Part model, mm, in its own coordinate system. Face numbers are marked on the shaded views. Coordinates: 2 decimals unless noted, no trailing zeros. Order: outer loops, then holes, each group sorted by start corner. A loop starts at its lowest first (then second) coordinate and runs counter-clockwise, first axis right, second up.
1) Cut at C-C (z = 6). List the corners of the cut face in (x, y), and give its area (3 significant figures).
2) Wall check: L1, parallel to Y at x = -13.25, z = 13; L2, parallel to X at y = 0, z = 9.5; L3, parallel to X at y = 1.5, z = 3. Give the ranges that are in metal, low to high.
3) Cut at A-A (x = -25.25). List the corners of the cut face in (y, z).
4) Cut at D-D (x = -12.25). List the corners of the cut face in (y, z).
5) Cut at B-B (z = 0.5). List the corners of the cut face in (x, y).
6) Mould opens along X. For the marked faces 1, 2 and 3 say: +X half, -X half, draft (parallel to the pull), parting line (faces both ways), or undercut.
7) Pin check, flat tips, straight feed: pin 1 Ø1 at (x, z) = (-10, 6.5) entering from -Y; pin 2 Ø6 at (x, y) = (-22.5, 7) entering from -Z; pin 3 Ø1 at (y, z) = (-4, -2) entering from -X. Stop position of each tip, or through.
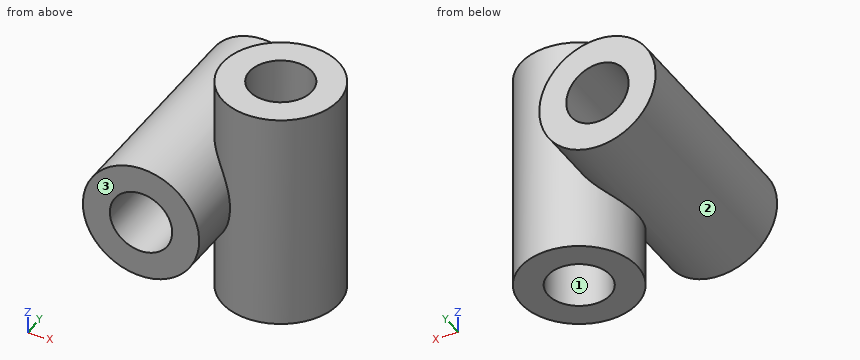
```python
from build123d import *

# Parameters (mm, degrees)
SKETCH1_R           = 28
SKETCH1_R_2         = 15
BOSS_EXTRUDE1_DEPTH = 53
SKETCH2_R           = 28
SKETCH2_R_2         = 15
BOSS_EXTRUDE2_DEPTH = 53
SKETCH3_R           = 15
CUT_EXTRUDE1_DEPTH  = 136.650285827
SCALE1_SCALE        = 0.3


with BuildPart() as part:
    # Sketch1 → Boss-Extrude1 (new, symmetric)
    with BuildSketch(Plane.XY):
        Circle(SKETCH1_R)
        Circle(SKETCH1_R_2, mode=Mode.SUBTRACT)
    extrude(amount=BOSS_EXTRUDE1_DEPTH, both=True)

    # Sketch2 → Boss-Extrude2 (add, symmetric)
    with BuildSketch(Plane(origin=(0, 0, 0), x_dir=(1, 0, 0), z_dir=(0, 1, 0))):
        with Locations(Location((-38, 0, 0), (0, 0, 270))):
            Circle(SKETCH2_R)
        with Locations(Location((-38, 0, 0), (0, 0, 270))):
            Circle(SKETCH2_R_2, mode=Mode.SUBTRACT)
    extrude(amount=BOSS_EXTRUDE2_DEPTH, both=True)

    # Sketch3 → Cut-Extrude1 (cut, through all)
    with BuildSketch(Plane(origin=(0, 53, 0), x_dir=(1, 0, 0), z_dir=(0, 1, 0))):
        with Locations(Location((-38, 0, 0), (0, 0, 270))):
            Circle(SKETCH3_R)
    extrude(amount=-CUT_EXTRUDE1_DEPTH, mode=Mode.SUBTRACT)


with BuildPart() as part_1:
    # Scale1: scaled about (-18.971831543, 0.000154548, 3.0881e-05)
    add(part.part.scale(SCALE1_SCALE).moved(Location((-13.28028208, 0.000108184, 2.1617e-05))))


solid = part_1.part
```
Geometry check:
1. outline: (-30.56, -15.9) - (-18.8, -15.9) - (-18.8, -6.33) arc R8.4 ccw (long way) to (-18.8, 6.33) - (-18.8, 15.9) - (-30.56, 15.9) - close; hole circle Ø9 at (-13.28, 0)
1. area: 507 mm2
2. L1: y = -8.4 to -4.5, 4.5 to 8.4
2. L2: x = -21.68 to -17.78, -8.78 to -4.88
2. L3: x = -32.53 to -28.03, -21.33 to -16.83, -9.04 to -5.02
3. outline: (-15.9, -8.38) - (15.9, -8.38) - (15.9, -4.46) - (-15.9, -4.46) - close; (-15.9, 4.46) - (15.9, 4.46) - (15.9, 8.38) - (-15.9, 8.38) - close
4. outline: (-8.34, -15.9) - (-4.38, -15.9) - (-4.38, 15.9) - (-8.34, 15.9) - close; (4.38, -15.9) - (8.34, -15.9) - (8.34, 15.9) - (4.38, 15.9) - close
5. outline: (-33.07, -15.9) - (-29.15, -15.9) - (-29.15, 15.9) - (-33.07, 15.9) - close; (-20.21, -15.9) - (-16.3, -15.9) - (-16.3, -7.84) arc R8.4 ccw (long way) to (-16.3, 7.84) - (-16.3, 15.9) - (-20.21, 15.9) - close; hole (-16.3, -3.34) arc R4.5 ccw (long way) to (-16.3, 3.34) - close
6. face 1: undercut
6. face 2: undercut
6. face 3: draft
7. pin 1: stops at y = -7.93
7. pin 2: stops at z = -8.4
7. pin 3: stops at x = -32.95
